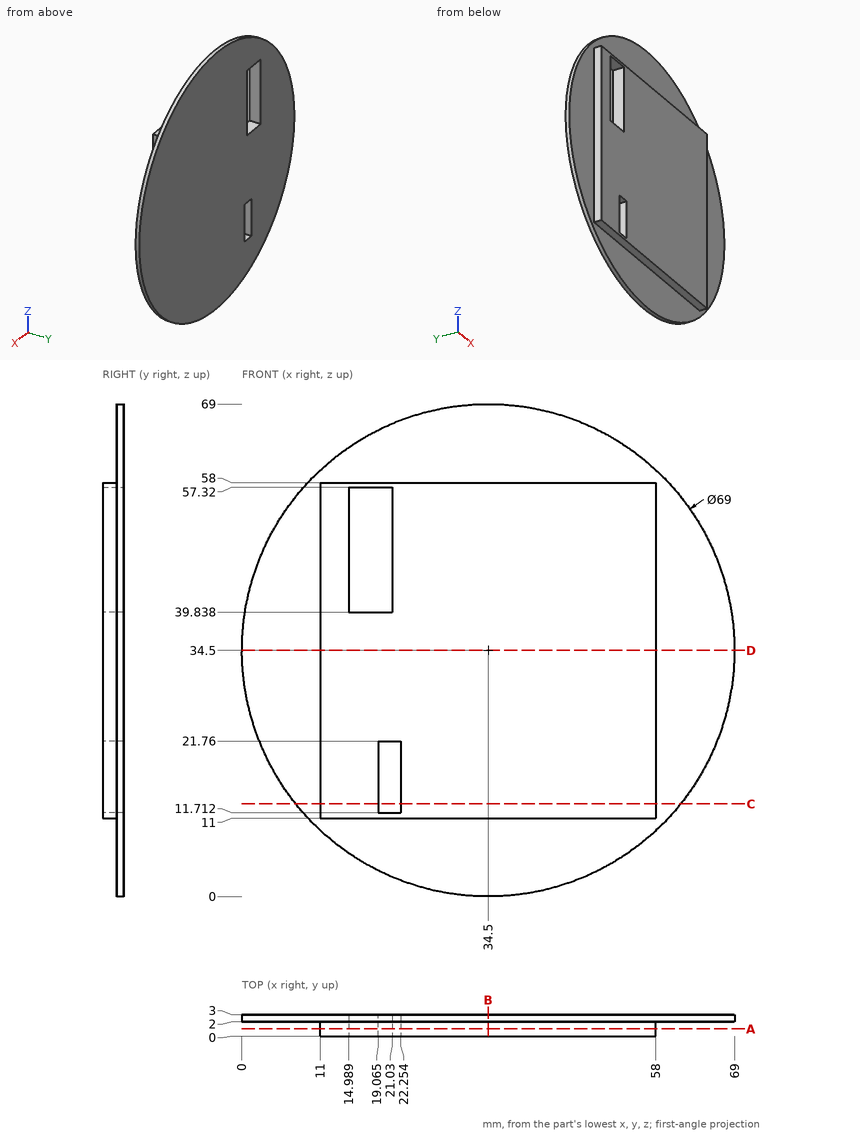
Geometry: see drawing. Coordinates: mm, zero at the bounding-box minimum. Give positions to 0.01 mm unless a question says otherwise; leave off trailing zeros. Loops run counter-clockwise (first coordinate to the right, second up) from the corner with the lowest first, then second, coordinate; pieces in that order, holes last. Notation, with made-up numbers: (77.25, -35.5) - (120.25, -35.5) arc R10 cw to (120.25, -28.5) - close; hole circle Ø11 at (67.25, 63.25). An arc over 180 degrees is marked (long way). Use CSV: the item, a comma, the result in double quotes. Start each with the question number.
Item 1: Section C-C on z = 13. Return loops of the section in (x, y) (1 decimal), then the cut area to 3 significant figures.
Item 2: Section A-A on y = 1. Return loops of the section in (x, z) (1 decimal).
Item 3: Contact query for flat-ended pins moving along their axis: P1, Ø1.6, axis at x = 26, y = 1.5, coming from the -Z side; P2, Ø0.9, axis at x = 21, y = 1, coming from the +Z side; P3, Ø1.5, axis at x = 21, y = 2, coming from the +Z side. Output: stop coordinate, or through.
Item 4: Section B-B on x = 34.5. Return loops of the section in (y, z), then the cut area to 3 significant figures.
Item 5: Section D-D on z = 34.5. Return loops of the section in (x, y), then the cut area to 3 significant figures.
Item 6: Line query: line 1 (X direction, y = 1.85, z = 14) (1 decimal); line 2 (X direction, y = 0.2, z = 46); line 3 (Y direction, x = 28, z = 59). Output: solid intervals per line, ascending.
Ans:
1,outline,"(7.5, 2) - (11, 2) - (11, 0) - (19.1, 0) - (19.1, 3) - (7.5, 3) - close; (22.3, 0) - (58, 0) - (58, 2) - (61.5, 2) - (61.5, 3) - (22.3, 3) - close"
1,area,"138 mm2"
2,outline,"(11, 11) - (58, 11) - (58, 58) - (11, 58) - close; hole (15, 39.8) - (21, 39.8) - (21, 57.3) - (15, 57.3) - close; hole (19.1, 11.7) - (22.3, 11.7) - (22.3, 21.8) - (19.1, 21.8) - close"
3,P1,"stops at z = 0.91"
3,P2,"stops at z = 58"
3,P3,"stops at z = 66.56"
4,outline,"(0, 11) - (2, 11) - (2, 0) - (3, 0) - (3, 69) - (2, 69) - (2, 58) - (0, 58) - close"
4,area,"163 mm2"
5,outline,"(0, 2) - (11, 2) - (11, 0) - (58, 0) - (58, 2) - (69, 2) - (69, 3) - (0, 3) - close"
5,area,"163 mm2"
6,line 1,"x = 11 to 19.1, 22.3 to 58"
6,line 2,"x = 11 to 14.99, 21.03 to 58"
6,line 3,"y = 2 to 3"
